CAD build for the part. Positions are in the model's coordinates, mm. Round coordinates to 2 decimals unless told otherwise and drop trailing zeros. Loops run counter-clockwise (first coordinate to the right, second up) from the corner with the lowest first, then second, coordinate; pieces in that order, holes last.
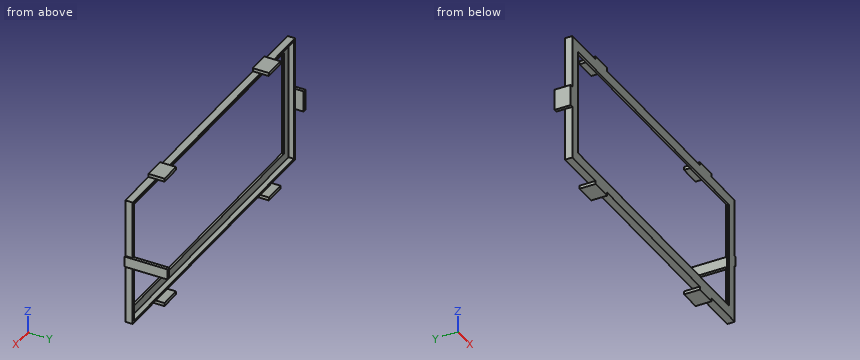
from build123d import *

# Parameters (mm, degrees)
SKETCH1_W           = 280
SKETCH1_H           = 120
BOSS_EXTRUDE1_DEPTH = 2
SKETCH2_W           = 280
SKETCH2_H           = 120
SKETCH2_W_2         = 276
SKETCH2_H_2         = 116
BOSS_EXTRUDE2_DEPTH = 5
SKETCH4_W           = 20
SKETCH4_H           = 3
SKETCH4_W_2         = 3
SKETCH4_H_2         = 20
BOSS_EXTRUDE3_DEPTH = 15
SKETCH5_W           = 3
SKETCH5_H           = 10
BOSS_EXTRUDE4_DEPTH = 40
SKETCH6_W           = 260
SKETCH6_H           = 100
CUT_EXTRUDE2_DEPTH  = 41


with BuildPart() as part:
    # Sketch1 → Boss-Extrude1 (new body)
    with BuildSketch(Plane(origin=(0, 0, 0), x_dir=(1, 0, 0), z_dir=(0, 1, 0))):
        with Locations((140, -60)):
            Rectangle(SKETCH1_W, SKETCH1_H)
    extrude(amount=BOSS_EXTRUDE1_DEPTH)

    # Sketch2 → Boss-Extrude2 (add)
    with BuildSketch(Plane(origin=(0, 2, 0), x_dir=(1, 0, 0), z_dir=(0, 1, 0))):
        with Locations((140, -60)):
            Rectangle(SKETCH2_W, SKETCH2_H)
        with Locations((140, -60)):
            Rectangle(SKETCH2_W_2, SKETCH2_H_2, mode=Mode.SUBTRACT)
    extrude(amount=BOSS_EXTRUDE2_DEPTH)

    # Sketch4 → Boss-Extrude3 (add)
    with BuildSketch(Plane(origin=(0, 0, 0), x_dir=(-1, 0, 0), z_dir=(0, -1, 0))):
        with Locations((-50, 1.5)):
            Rectangle(SKETCH4_W, SKETCH4_H)
        with Locations((-230, 1.5)):
            Rectangle(SKETCH4_W, SKETCH4_H)
        with Locations((-230, -121.5)):
            Rectangle(SKETCH4_W, SKETCH4_H)
        with Locations((-50, -121.5)):
            Rectangle(SKETCH4_W, SKETCH4_H)
        with Locations((1.5, -60)):
            Rectangle(SKETCH4_W_2, SKETCH4_H_2)
    extrude(amount=-BOSS_EXTRUDE3_DEPTH)

    # Sketch5 → Boss-Extrude4 (add)
    with BuildSketch(Plane(origin=(0, 0, 0), x_dir=(-1, 0, 0), z_dir=(0, -1, 0))):
        with Locations((-279.5, -60)):
            Rectangle(SKETCH5_W, SKETCH5_H)
    extrude(amount=-BOSS_EXTRUDE4_DEPTH)

    # Sketch6 → Cut-Extrude2 (cut, through all)
    with BuildSketch(Plane(origin=(0, 0, 0), x_dir=(-1, 0, 0), z_dir=(0, -1, 0))):
        with Locations((-140, -60)):
            Rectangle(SKETCH6_W, SKETCH6_H)
    extrude(amount=-CUT_EXTRUDE2_DEPTH, mode=Mode.SUBTRACT)


solid = part.part
Item 1: Cut at D-D (y = 37). List the corners of the cut face in (x, z), plus the area to 3 significant figures.
Verdict:
outline: (278, 55) - (281, 55) - (281, 65) - (278, 65) - close
area: 30.0 mm2
Item 2: Flat gauge pins, fed straight in: P1, Ø3.5, axis at x = 158, y = 3, coming from the +Z side; P2, Ø2.5, axis at y = 6.5, z = -1, coming from the -X side; P3, Ø2, axis at y = 5, z = 81, coming from the +X side. Where does each tip first touch, or does it go through?
Verdict:
P1: stops at z = 120
P2: stops at x = 0
P3: stops at x = 280
Item 3: Cut at B-B (x = 188). List the corners of the cut face in (y, z), plus the area to 3 significant figures.
Verdict:
outline: (0, 0) - (7, 0) - (7, 2) - (2, 2) - (2, 10) - (0, 10) - close; (0, 110) - (2, 110) - (2, 118) - (7, 118) - (7, 120) - (0, 120) - close
area: 60.0 mm2
Item 4: Wall check: L1, parallel to X at y = 4.5, z = 48.5; L2, parallel to Z at x = 59.5, y = 3.5; L3, parallel to X at y = 12, z = 56. Give the ranges that are in metal, low to high.
Verdict:
L1: x = 0 to 2, 278 to 280
L2: z = -3 to 2, 118 to 123
L3: x = -3 to 0, 278 to 281
Item 5: Cut at A-A (z = 25.5). List the corners of the cut face in (x, y).
Verdict:
outline: (0, 0) - (10, 0) - (10, 2) - (2, 2) - (2, 7) - (0, 7) - close; (270, 0) - (280, 0) - (280, 7) - (278, 7) - (278, 2) - (270, 2) - close
Item 6: Cut at C-C (z = 114.5). List the corners of the cut face in (x, y).
Verdict:
outline: (0, 0) - (280, 0) - (280, 7) - (278, 7) - (278, 2) - (2, 2) - (2, 7) - (0, 7) - close
